```python
from build123d import *

# Parameters (mm, degrees)
SKETCH_1_W          = 80
SKETCH_1_H          = 40
SKETCH_1_W_2        = 76
SKETCH_1_H_2        = 36
EXTRUDE_1_DEPTH     = 72
CUT_EXTRUDE_1_DEPTH = 73


with BuildPart() as part:
    # Эскиз1 → Бобышка-Вытянуть1 (new body)
    with BuildSketch(Plane.XY):
        Rectangle(SKETCH_1_W, SKETCH_1_H)
        Rectangle(SKETCH_1_W_2, SKETCH_1_H_2, mode=Mode.SUBTRACT)
    extrude(amount=EXTRUDE_1_DEPTH)

    # Эскиз2 → Вырез-Вытянуть1 (cut, through all)
    with BuildSketch(Plane.XY.offset(72)):
        Polygon((-40, 20), (-40, 9), (-38, 9), (-38, 18), (38, 18), (38, -18), (14, -18), (14, -20), (40, -20), (40, 20), align=None)
    extrude(amount=-CUT_EXTRUDE_1_DEPTH, mode=Mode.SUBTRACT)


solid = part.part
```
Verification items for the finished model (mm, model axes). A direction names the side the tool comes from. Coordinates: 2 decimals unless noted, no trailing zeros. Loops run counter-clockwise (first coordinate to the right, second up) from the corner with the lowest first, then second, coordinate; pieces in that order, holes last. Notation, with made-up numbers: (40.5, -32) -> (52.5, -32) arc R12 cw to (52.5, -28) -> close; hole circle Ø7 at (10, -37.75). An arc over 180 degrees is marked (long way). Answer in a Markdown table with one row per item. Add a question column.
1. Section check B-B, the plane y = -9.5. Enter the section's corners in (x, z).
2. Section check A-A, the plane z = 9. Enter the section's corners in (x, y).
3. Section check C-C, the plane x = -10. Enter the section's corners in (y, z), then the cut area to 3 significant figures.
4. Material ranges on probe 1 along Y at (x, z) = (-31, 37); probe 2 along X at (y, z) = (-3.5, 7), recorded low to high. Write a range as [from, to].
5. Depth check by flat-ended pin: P1, Ø10, axis at y = 5, z = 22, coming from the +X side; P2, Ø12, axis at x = -11, y = -10.5, coming from the -Z side; P3, Ø2, axis at x = -20, z = 10, coming from the +Y side. Enter the tip coordinate at first touch or a pass-through.
6. Access from +Z, -Z, +X, -X, +Y, -Y to the whole of each face (thin tool, end or side, straight path). Record for faces 1 (the face through (-38, -5, 35)), 2 (the face through (-40, -6, 35)).
Derived:
| question | item | result |
|---|---|---|
| 1 | outline | (-40, 0) -> (-38, 0) -> (-38, 72) -> (-40, 72) -> close |
| 2 | outline | (-40, -20) -> (14, -20) -> (14, -18) -> (-38, -18) -> (-38, 9) -> (-40, 9) -> close |
| 3 | outline | (-20, 0) -> (-18, 0) -> (-18, 72) -> (-20, 72) -> close |
| 3 | area | 144 mm² |
| 4 | probe 1 | y = [-20, -18] |
| 4 | probe 2 | x = [-40, -38] |
| 5 | P1 | stops at x = -38 |
| 5 | P2 | passes through |
| 5 | P3 | stops at y = -18 |
| 6 | face 1 | +Z, -Z, +X, +Y |
| 6 | face 2 | +Z, -Z, -X, +Y, -Y |
